Build history of the part. All positions in model axes, mm. A direction names the side the tool comes from. Give positions to 0.01 mm unless a question says otherwise; leave off trailing zeros. Loops run counter-clockwise (first coordinate to the right, second up) from the corner with the lowest first, then second, coordinate; pieces in that order, holes last. Notation, with made-up numbers: (5.25, 33) -> (53.25, 33) arc R25 ccw to (53.25, 71) -> close; hole circle Ø4 at (88, 68.5). An arc over 180 degrees is marked (long way). One line per question, with ' | ' between items. Start each with the question number.
(1) 3-axis set-ups, long thin cutter, end or side, ignore diameter. For faces 5 (the face through (0, 15.526, 16)), 6 (the face through (1, -8.894, 17)): which of +Z, -Z, +X, -X, +Y, -Y reach the whole face in a straight line?
(2) Slice it at C-C, the plane x = 3.75. Write the cut outline in (y, z), then the cut area to 3 significant figures.
(3) Mould opens along X. For faces 1 (the face through (11.14, -9.83, 16.27)), 2 (the face through (-6.3, 4.2, 33)), 3 (the face through (-10.043, 11.103, 16.269)), 4 (the face through (3.147, -8, 17)) say: pulls with the +X half, pulls with the -X half, needs draft (parallel to the pull), parting line crosses it, or undercut.
(4) Slice it at D-D, the plane y = -11.25. Write the cut outline in (x, z), then the cut area to 3 significant figures.
(5) Flat gauge pins, fed straight in: pin 1 Ø12 at (x, y) = (0.55, 0.64) entering from +Z; pin 2 Ø2 at (y, z) = (-7.5, 9) entering from +X; pin 3 Ø6 at (x, z) = (-11.5, 10) entering from +Y; pin 4 Ø2.5 at (y, z) = (-8, 10) entering from -X. Where does each tip first touch, or does it go through?
(6) Drill centre lines: L1, parallel to Y at x = 1.75, z = 19; L2, parallel to X at y = -6, z = 23; L3, parallel to X at y = 5, z = 21.5. Where is each one in solid material? Low to high. Write a range as from..to.
(7) Slice it at A-A, the plane z = 5. Write the cut outline in (x, y).
(8) Slice it at B-B, the plane y = 6. Write the cut outline in (x, z), then the cut area to 3 significant figures.
Autodesk Inventor part; units mm, degrees
ref_plane "YZ Plane" through (0, 0, 0) normal (1, 0, 0) x (0, 1, 0)
ref_plane "XZ Plane" through (0, 0, 0) normal (0, 1, 0) x (-1, 0, 0)
ref_plane "XY Plane" through (0, 0, 0) normal (0, 0, 1) x (1, 0, 0)
sketch "Sketch1" plane through (0, 0, 0) normal (0, 0, 1) x (1, 0, 0)
  circle A0 centre (-19.4529, 0.6357) radius 3.1
  circle A1 centre (0.5471, -19.3643) radius 3.1
  circle A2 centre (20.5471, 0.6357) radius 3.1
  circle A3 centre (-13.595, 14.7778) radius 3.1
  line L0 (15.4871, -5.5527) -> (6.7355, -14.3043)
  line L1 (6.7355, -14.3043) -> (-5.6412, -14.3043)
  line L2 (-5.6412, -14.3043) -> (-14.3929, -5.5527)
  line L3 (-14.3929, -5.5527) -> (-14.3929, 6.824)
  line L4 (-14.3929, 6.824) -> (-5.6412, 15.5757)
  line L5 (-5.6412, 15.5757) -> (6.7355, 15.5757)
  line L6 (6.7355, 15.5757) -> (15.4871, 6.824)
  line L7 (15.4871, 6.824) -> (15.4871, -5.5527)
  circle A4 centre (14.6893, 14.7778) radius 3.1
  circle A5 centre (14.6893, -13.5064) radius 3.1
  circle A6 centre (-13.595, -13.5064) radius 3.1
  arc A7 (-10.3042, 22.9357) -> (11.3984, 22.9357) centre (0.5471, 0.6357) ccw
  line L8 (-10.3042, 22.9357) -> (11.3984, 22.9357)
  point P0 (0, 0)
extrude "Extrusion1" add sketch "Sketch1" along normal blind 33 contours L0 L1 L2 L3 L4 L5 L6 L7
sketch "Sketch2" plane through (0, 0, 33) normal (0, 0, 1) x (1, 0, 0)
  arc A0 (3.1471, -6.3992) -> (-2.0529, -6.3992) centre (0.5471, 0.6357) ccw
  line L0 (3.1471, -8.8943) -> (3.1471, -6.3992)
  line L1 (-2.0529, -8.8943) -> (3.1471, -8.8943)
  line L2 (-2.0529, -8.8943) -> (-2.0529, -6.3992)
  line L3 (0.5471, 0.6357) -> (-14.3929, 0.6357)
  line L4 (-14.3929, 6.824) -> (-14.3929, -5.5527)
  line L5 (0.5471, 0.6357) -> (15.4871, 0.6357)
  line L6 (15.4871, -5.5527) -> (15.4871, 6.824)
  line L7 (0.5471, 0.6357) -> (0.5471, 15.5757)
  line L8 (6.7355, 15.5757) -> (-5.6412, 15.5757)
  point P0 (0, 0)
  point P1 (0.5471, 0.6357)
  point P2 (1.7246, 0.9714)
  dimension "d2" = 7.5
  dimension "d3" = 5.2
  dimension "d4" = 2.4951
  dimension "d5" = 2.6
extrude "Extrusion2" cut sketch "Sketch2" against normal through all
thicken "Thicken1" operation cut thickness 0.05 both sides no extend neighbours no toward (0, -1, 0) faces at (2.6099, 15.5757, 11) (12.5699, 9.7413, 22) (15.4871, -1.4271, 11) (9.6527, -11.3871, 11) (-1.5157, -14.3043, 11) (-11.4757, -8.4699, 11) (-14.3929, 2.6985, 11) (-8.5585, 12.6585, 11)
sketch "Sketch3" plane through (0, 0, 33) normal (0, 0, 1) x (1, 0, 0)
  line L0 (6.7148, -14.2543) -> (15.4371, -5.5319)
  line L1 (15.4371, -5.5319) -> (15.4371, 6.8033)
  line L2 (15.4371, 6.8033) -> (6.7148, 15.5257)
  line L3 (6.7148, 15.5257) -> (-5.6205, 15.5257)
  line L4 (-5.6205, 15.5257) -> (-14.3429, 6.8033)
  line L5 (-14.3429, 6.8033) -> (-14.3429, -5.5319)
  line L6 (-14.3429, -5.5319) -> (-5.6205, -14.2543)
  line L7 (-5.6205, -14.2543) -> (6.7148, -14.2543)
  line L8 (-2.0529, -8.8943) -> (-2.0529, -6.3992)
  arc A0 (3.1471, -6.3992) -> (-2.0529, -6.3992) centre (0.5471, 0.6357) ccw
  line L9 (3.1471, -6.3992) -> (3.1471, -8.8943)
  line L10 (3.1471, -8.8943) -> (-2.0529, -8.8943)
  point P0 (0, 0)
properties part number "spool_keyway"
Final values:
1) face 5: +Z, -Z, +X, -X, +Y | face 6: +Z, -Z
2) outline: (-14.25, 0) -> (-6.15, 0) -> (-6.15, 33) -> (-14.25, 33) -> close; (7.42, 0) -> (15.53, 0) -> (15.53, 33) -> (7.42, 33) -> close | area: 535 mm2
3) face 1: pulls with the +X half | face 2: needs draft | face 3: pulls with the -X half | face 4: undercut
4) outline: (-8.62, 0) -> (9.72, 0) -> (9.72, 33) -> (-8.62, 33) -> close | area: 605 mm2
5) pin 1: through | pin 2: x = 14.47 | pin 3: y = 12.65 | pin 4: x = -13.12
6) L1: -14.25..-8.89, 8.04..15.53 | L2: -13.87..-2.95, 4.04..14.97 | L3: -14.34..-5.55, 6.65..15.44
7) outline: (-14.34, -5.53) -> (-5.62, -14.25) -> (6.71, -14.25) -> (15.44, -5.53) -> (15.44, 6.8) -> (6.71, 15.53) -> (-5.62, 15.53) -> (-14.34, 6.8) -> close; hole (-2.05, -8.89) -> (3.15, -8.89) -> (3.15, -6.4) arc R7.5 ccw (long way) to (-2.05, -6.4) -> close
8) outline: (-14.34, 0) -> (-4.69, 0) -> (-4.69, 33) -> (-14.34, 33) -> close; (5.79, 0) -> (15.44, 0) -> (15.44, 33) -> (5.79, 33) -> close | area: 637 mm2
